Design review of the part shown in the three views and the two pictorial views. Dimensions are in mm from the part's minimum x, y and z. A direction names the side the tool comes from. Give positions to 0.01 mm unless a question says otherwise; leave off trailing zeros. Loops run counter-clockwise (first coordinate to the right, second up) from the corner with the lowest first, then second, coordinate; pieces in that order, holes last. Notation, with made-up numbers: (81.5, 85.5) -> (109.5, 85.5) arc R11 cw to (109.5, 98.5) -> close; hole circle Ø8 at (-31.75, 18.25). An arc over 180 degrees is marked (long way). Use CSV: the item, a comma, the result in double quotes. Start each with the question number.
Item 1: We need section B-B (y = 28). State the section outline as (x, z) points, plus the area to 3 significant figures.
Item 2: For the marked faces 1, 2, 3, 4 and 5, list the 3-axis set-ups (+Z, -Z, +X, -X, +Y, -Y) from which the entire face can be reached by the end or side of a thin tool; tool diameter is ignored.
Item 3: Clearance check with flat-ended pins moving along their axes: pin 1 (9.5 mm diameter, centred on x = 15.5, z = 20.5, fed in from -Y); pin 2 (3 mm diameter, centred on x = 30.5, y = 35, fed in from +Z); pin 3 (8 mm diameter, centred on y = 32.5, z = 22.5, fed in from +X) (1 decimal). State where each tip first meets the part, or that it passes through.
Item 4: Wall thickness on line 1 along Y through (x, z) = (9.5, 24.5); line 2 along X through (y, z) = (33.5, 29); line 3 along Z through (x, y) = (6.5, 36.5): over which ranges is each line inside the solid? List them lowest first. Write a range as from..to.
Item 5: We need section C-C (z = 26). State the section outline as (x, y) points, plus the area to 3 significant figures.
Item 6: We need section A-A (z = 18). State the section outline as (x, y) points, plus the area to 3 significant figures.
Item 7: We need section D-D (x = 16.5). State the section outline as (y, z) points.
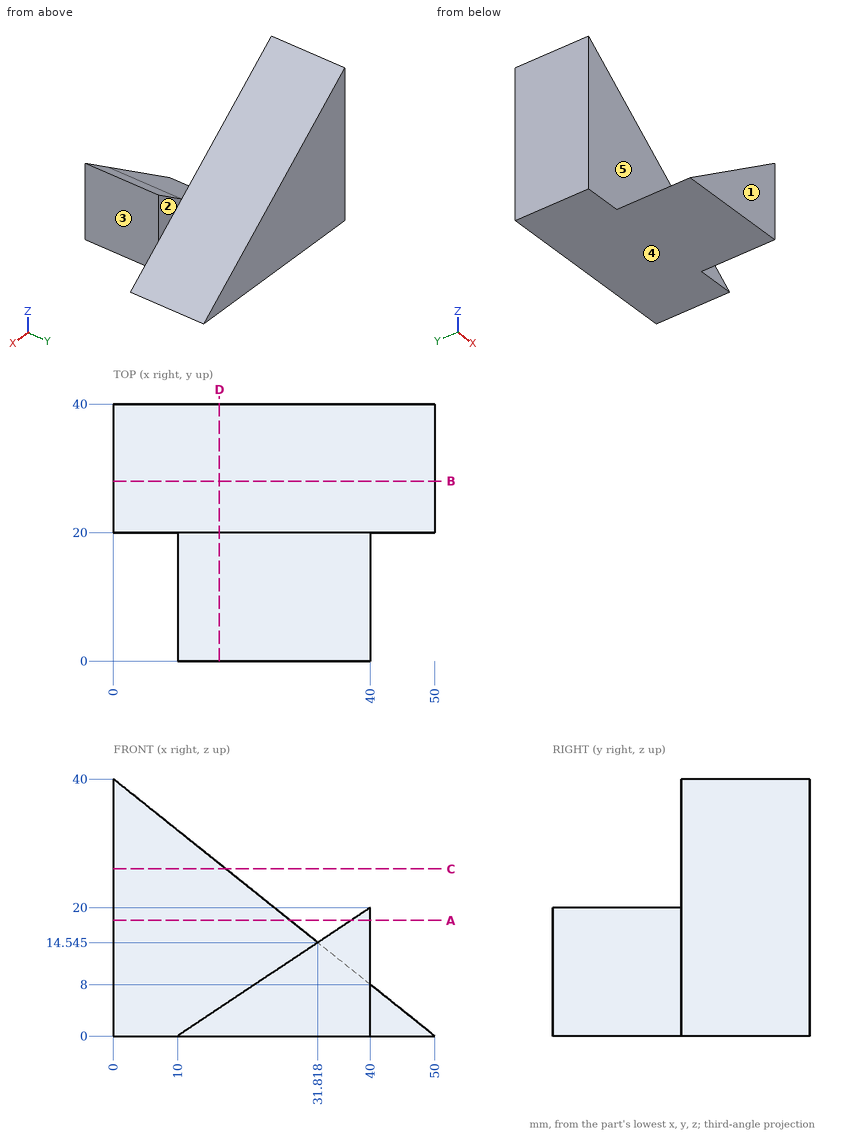
Results found:
1,outline,"(0, 0) -> (50, 0) -> (0, 40) -> close"
1,area,"1,000 mm²"
2,face 1,"+Z, -Z, +X, -X, -Y"
2,face 2,"+Z, +X, +Y"
2,face 3,"+Z, -Z, +X, -Y"
2,face 4,"-Z, +X, -X, +Y, -Y"
2,face 5,"+Z, -X, -Y"
3,pin 1,"y = 20"
3,pin 2,"z = 16.8"
3,pin 3,"x = 26.9"
4,line 1,"20..40"
4,line 2,"0..13.75"
4,line 3,"0..34.8"
5,outline,"(0, 20) -> (17.5, 20) -> (17.5, 40) -> (0, 40) -> close"
5,area,"350 mm²"
6,outline,"(0, 20) -> (27.5, 20) -> (27.5, 40) -> (0, 40) -> close; (37, 0) -> (40, 0) -> (40, 20) -> (37, 20) -> close"
6,area,"610 mm²"
7,outline,"(0, 0) -> (40, 0) -> (40, 26.8) -> (20, 26.8) -> (20, 4.33) -> (0, 4.33) -> close"
